```python
from build123d import *

# Parameters (mm, degrees)
EXTRUDE_1_DEPTH          = 2.5
FILLET_2_R               = 10
FILLET_3_R               = 3
SKETCH_2_R               = 31
CUT_EXTRUDE_1_DEPTH      = 1
CUT_EXTRUDE_1_DEPTH_BACK = 6
SKETCH_3_R               = 1.525
CUT_EXTRUDE_2_DEPTH      = 1
CUT_EXTRUDE_2_DEPTH_BACK = 6
SKETCH_4_R               = 2.025
CUT_EXTRUDE_3_DEPTH      = 6
EXTRUDE_2_DEPTH          = 5
FILLET_4_R               = 3
SKETCH_8_R               = 1.525
CUT_EXTRUDE_6_DEPTH      = 10
SKETCH_9_W               = 20
SKETCH_9_H               = 5
EXTRUDE_3_DEPTH          = 5
CUT_EXTRUDE_7_DEPTH      = 14
SKETCH_11_W              = 5
SKETCH_11_H              = 25
EXTRUDE_4_DEPTH          = 5
CUT_EXTRUDE_8_DEPTH      = 5
SKETCH_13_R              = 1.525
CUT_EXTRUDE_9_DEPTH      = 6


with BuildPart() as part:
    # 草图1 → 凸台-拉伸1 (new body, symmetric)
    with BuildSketch(Plane.XY):
        with BuildLine():
            Line((80, 47.5), (80, -47.5))
            Line((80, -47.5), (15, -47.5))
            Line((15, -47.5), (-10.218604944, -41.253243666))
            ThreePointArc((-10.218604944, -41.253243666), (-42.5, 0), (-10.218604944, 41.253243666))
            Line((-10.218604944, 41.253243666), (15, 47.5))
            Line((15, 47.5), (80, 47.5))
        make_face()
    extrude(amount=EXTRUDE_1_DEPTH, both=True)

    # 圆角2
    fillet_2_edges = [part.edges().sort_by_distance(p)[0] for p in [
        (15, -47.5, 0),
        (15, 47.5, 0),
    ]]
    fillet(fillet_2_edges, radius=FILLET_2_R)

    # 圆角3
    fillet_3_edges = [part.edges().sort_by_distance(p)[0] for p in [
        (80, 47.5, 0),
        (80, -47.5, 0),
    ]]
    fillet(fillet_3_edges, radius=FILLET_3_R)

    # 草图2 → 切除-拉伸1 (cut, two sides)
    with BuildSketch(Plane(origin=(0, 0, -2.5), x_dir=(-1, 0, 0), z_dir=(0, 0, -1))) as cut_extrude_1_sk:
        Circle(SKETCH_2_R)
    extrude(amount=CUT_EXTRUDE_1_DEPTH, mode=Mode.SUBTRACT)
    extrude(cut_extrude_1_sk.sketch, amount=-CUT_EXTRUDE_1_DEPTH_BACK, mode=Mode.SUBTRACT)

    # 草图3 → 切除-拉伸2 (cut, two sides)
    with BuildSketch(Plane.XY.offset(2.5)) as cut_extrude_2_sk:
        with Locations((9.576304669, 35.739255573)):
            Circle(SKETCH_3_R)
        with Locations((26.162950904, 26.162950904)):
            Circle(SKETCH_3_R)
        with Locations((35.739255573, 9.576304669)):
            Circle(SKETCH_3_R)
        with Locations((35.739255573, -9.576304669)):
            Circle(SKETCH_3_R)
        with Locations((26.162950904, -26.162950904)):
            Circle(SKETCH_3_R)
        with Locations((9.576304669, -35.739255573)):
            Circle(SKETCH_3_R)
        with Locations((-9.576304669, -35.739255573)):
            Circle(SKETCH_3_R)
        with Locations((-26.162950904, -26.162950904)):
            Circle(SKETCH_3_R)
        with Locations((-35.739255573, -9.576304669)):
            Circle(SKETCH_3_R)
        with Locations((-35.739255573, 9.576304669)):
            Circle(SKETCH_3_R)
        with Locations((-26.162950904, 26.162950904)):
            Circle(SKETCH_3_R)
        with Locations((-9.576304669, 35.739255573)):
            Circle(SKETCH_3_R)
    extrude(amount=CUT_EXTRUDE_2_DEPTH, mode=Mode.SUBTRACT)
    extrude(cut_extrude_2_sk.sketch, amount=-CUT_EXTRUDE_2_DEPTH_BACK, mode=Mode.SUBTRACT)

    # 草图4 → 切除-拉伸3 (cut, through all)
    with BuildSketch(Plane.XY.offset(2.5)):
        with Locations((76, -33.5)):
            Circle(SKETCH_4_R)
        with Locations((76, -18.5)):
            Circle(SKETCH_4_R)
        with Locations((76, 18.5)):
            Circle(SKETCH_4_R)
        with Locations((76, 33.5)):
            Circle(SKETCH_4_R)
    extrude(amount=-CUT_EXTRUDE_3_DEPTH, mode=Mode.SUBTRACT)

    # 草图6 → 凸台-拉伸2 (add)
    with BuildSketch(Plane.XY.offset(2.5)):
        with BuildLine():
            Line((-15, 44.5), (-15, 39.764934301))
            Line((-15, 39.764934301), (16.220084679, 47.5))
            Line((16.220084679, 47.5), (-12, 47.5))
            ThreePointArc((-12, 47.5), (-14.121320344, 46.621320344), (-15, 44.5))
        make_face()
    extrude_2 = extrude(amount=-EXTRUDE_2_DEPTH)

    # 镜向1: 凸台-拉伸2 across plane
    add(extrude_2.mirror(Plane.ZX))

    # 圆角4
    fillet_4_edges = [part.edges().sort_by_distance(p)[0] for p in [
        (-15, 39.764934301, 0),
        (-15, -39.764934301, 0),
    ]]
    fillet(fillet_4_edges, radius=FILLET_4_R)

    # 草图8 → 切除-拉伸6 (cut)
    with BuildSketch(Plane.XY.offset(2.5)):
        with Locations((66.03743584, 44.5)):
            Circle(SKETCH_8_R)
        with Locations((46.03743584, 44.5)):
            Circle(SKETCH_8_R)
    cut_extrude_6 = extrude(amount=-CUT_EXTRUDE_6_DEPTH, mode=Mode.SUBTRACT)

    # 草图9 → 凸台-拉伸3 (add)
    with BuildSketch(Plane(origin=(0, 47.5, 0), x_dir=(1, 0, 0), z_dir=(0, 1, 0))):
        with Locations((52, 0)):
            Rectangle(SKETCH_9_W, SKETCH_9_H)
    extrude_3 = extrude(amount=EXTRUDE_3_DEPTH)

    # 草图10 → 切除-拉伸7 (cut)
    with BuildSketch(Plane.XY.offset(2.5)):
        with BuildLine():
            Line((39.9, 47.5), (42, 47.5))
            ThreePointArc((42, 47.5), (40.95, 46.45), (39.9, 47.5))
        make_face()
        with BuildLine():
            Line((62, 47.5), (64.1, 47.5))
            ThreePointArc((64.1, 47.5), (63.05, 46.45), (62, 47.5))
        make_face()
    cut_extrude_7 = extrude(amount=-CUT_EXTRUDE_7_DEPTH, mode=Mode.SUBTRACT)

    # 镜向3: 切除-拉伸6, 凸台-拉伸3 across plane
    add(cut_extrude_6.mirror(Plane.ZX), mode=Mode.SUBTRACT)
    add(extrude_3.mirror(Plane.ZX))

    # 草图11 → 凸台-拉伸4 (add)
    with BuildSketch(Plane(origin=(80, 0, 0), x_dir=(0, 0, -1), z_dir=(1, 0, 0))):
        with Locations((0, 26)):
            Rectangle(SKETCH_11_W, SKETCH_11_H)
    extrude_4 = extrude(amount=EXTRUDE_4_DEPTH)

    # 草图12 → 切除-拉伸8 (cut)
    with BuildSketch(Plane.XY.offset(2.5)):
        with BuildLine():
            Line((80, 11.4), (80, 13.5))
            ThreePointArc((80, 13.5), (78.95, 12.45), (80, 11.4))
        make_face()
        with BuildLine():
            Line((80, 40.6), (80, 38.5))
            ThreePointArc((80, 38.5), (78.95, 39.55), (80, 40.6))
        make_face()
    cut_extrude_8 = extrude(amount=-CUT_EXTRUDE_8_DEPTH, mode=Mode.SUBTRACT)

    # 镜向4: 凸台-拉伸4, 切除-拉伸8 across plane
    add(extrude_4.mirror(Plane.ZX))
    add(cut_extrude_8.mirror(Plane.ZX), mode=Mode.SUBTRACT)

    # 草图13 → 切除-拉伸9 (cut, through all)
    with BuildSketch(Plane.XY.offset(2.5)):
        with Locations((59, 9)):
            Circle(SKETCH_13_R)
        with Locations((59, 24)):
            Circle(SKETCH_13_R)
    cut_extrude_9 = extrude(amount=-CUT_EXTRUDE_9_DEPTH, mode=Mode.SUBTRACT)

    # 镜向5: 切除-拉伸9 across plane
    add(cut_extrude_9.mirror(Plane.ZX), mode=Mode.SUBTRACT)

    # 镜向6: 凸台-拉伸3, 切除-拉伸7 across plane
    add(extrude_3.mirror(Plane.ZX))
    add(cut_extrude_7.mirror(Plane.ZX), mode=Mode.SUBTRACT)


solid = part.part
```
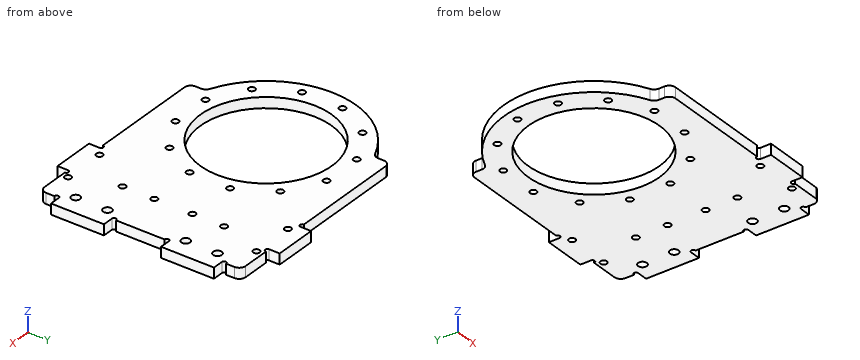
Read the model definition and answer for the solid it produces. Units are mm, in the model's axes. Round coordinates to 2 decimals unless told otherwise and drop trailing zeros. Write each loop counter-clockwise with the first axis right and the second up, starting at its lowest first coordinate (ties: lowest second). Pieces come first, ordered by that corner, then holes. Notation, with made-up numbers: M -37.5,59.5 L -28.5,59.5 A25 cw -28.5,84.5 Z; hole C 50,22 d6. An arc over 180 degrees is marked long. One line per item, written item: value.
Q1. Find section D-D on z = 1.25. Count the separate pieces of the cut face and the enclosed holes in it, plus the area to 3 significant figures.
Data:
separate pieces: 1
enclosed holes: 25
area: 7,830 mm2
Q2. Find section C-C on y = -18.5. Write down the section's boundary in (x, z) (3 decimals).
Data:
outline: M -38.262,-2.5 L -24.875,-2.5 L -24.875,2.5 L -38.262,2.5 Z; M 24.875,-2.5 L 73.975,-2.5 L 73.975,2.5 L 24.875,2.5 Z; M 78.025,-2.5 L 85,-2.5 L 85,2.5 L 78.025,2.5 Z
Q3. Find section A-A on x = 0. Write down the section's boundary in (y, z), plus the area to 3 significant figures.
Data:
outline: M -47.5,-2.5 L -31,-2.5 L -31,2.5 L -47.5,2.5 Z; M 31,-2.5 L 47.5,-2.5 L 47.5,2.5 L 31,2.5 Z
area: 165 mm2
Q4. Straight lines are drawn through the part: line 1 (Y direction, x = 46, z = -0.9); line 2 (Y direction, x = 59, z = -1.3) (3 decimals); line 3 (X direction, y = -9, z = 0.25) (3 decimals). For each, find the intervals that lie inside material, in ascending order. Write a range as [from, to].
Data:
line 1: [-52.5, -46.02], [-42.98, 42.98], [46.02, 52.5]
line 2: [-52.5, -25.525], [-22.475, -10.525], [-7.475, 7.475], [10.525, 22.475], [25.525, 52.5]
line 3: [-41.536, -37.151], [-34.327, -29.665], [29.665, 34.327], [37.151, 57.475], [60.525, 80]
Q5. Find section B-B on y = 0. Write down the section's boundary in (x, z), plus the area to 4 significant figures.
Data:
outline: M -42.5,-2.5 L -31,-2.5 L -31,2.5 L -42.5,2.5 Z; M 31,-2.5 L 80,-2.5 L 80,2.5 L 31,2.5 Z
area: 302.5 mm2
Q6. Flat-ended cylindrical pins translate along their axes: pin 1 Ø2.5 at (x, y) = (59, -24) entering from -Z; pin 2 Ø4 at (x, y) = (66.04, -44.5) entering from +Z; pin 3 Ø2.5 at (x, z) = (83, 0) entering from -Y; pin 4 Ø2 at (x, z) = (19, -0.5) entering from +Y. Find the tip coordinate at first contact, or state that the pin passes through.
Data:
pin 1: through
pin 2: z = 2.5
pin 3: y = -38.5
pin 4: y = 47.5
